Source: CAD feature listing. Evaluate the final solid. Frame: model axes, mm. A direction names the side the tool comes from. Round coordinates to 2 decimals unless told otherwise and drop trailing zeros. Loops run counter-clockwise (first coordinate to the right, second up) from the corner with the lowest first, then second, coordinate; pieces in that order, holes last.
Item 1: First-contact query: P1, Ø1, axis at y = 6, z = -2, coming from the -X side; P2, Ø2, axis at x = 20.5, y = 5, coming from the -Z side; P3, Ø10, axis at x = -63.5, y = 0, coming from the -Z side; P4, Ø1, axis at y = -1, z = 3.5, coming from the +X side. Flat tips, straight axial feed; report the tip coordinate or a pass-through.
Item 2: Section query C-C on x = -6. Return loops of the section in (y, z), then the cut area to 3 significant figures.
Item 3: Section query B-B on y = 3. Give the number of separate pieces and of enclosed holes in the cut face, then the cut area to 3 significant figures.
Item 4: Section query A-A on x = 67.5. Return loops of the section in (y, z), then the cut area to 3 significant figures.
Item 5: Pull-direction query (Y, two-part tool) for faces 3 (the cylindrical face through (-57.54, 1.88, -2.58)), 4 (the flat face through (-1, -12.7, 2)), 5 (the flat face through (-66.8, -5.5, 0)); classes: released by +Y, released by -Y, zero draft, split by the parting line, or undercut.
Item 6: Ray query, L1, parallel to Y at x = -63.5, z = -1.15; L2, parallel to Z at x = -1, y = -2.25; L3, parallel to X at y = 4.25, z = -3.25. Return the intervals inside material, ascending.
Item 7: Access query for faces 1 (the flat face through (1, 12.7, 2)), 2 (the flat face through (16, 0, 0)). Directions: +Z, -Z, +X, -X, +Y, -Y. A direction counts if a zero-diameter tool reaches every point of the face in a straight line with its end or side. Return the directions, or none.
```python
from build123d import *

# Parameters (mm, degrees)
SKETCH1_W                    = 152.4
SKETCH1_H                    = 25.4
BOSS_EXTRUDE1_DEPTH          = 5.08
F_12_5_12_5_DIAMETER_HOLE1_D = 12.5
FILLET3_R                    = 12.7
CUT_EXTRUDE1_START           = -76.2
CUT_EXTRUDE1_OUTLINE_W       = 25.4
CUT_EXTRUDE1_OUTLINE_H       = 2.54
CUT_EXTRUDE1_DEPTH           = 28.395084053
BOSS_EXTRUDE2_START          = -7.62
SKETCH10_R                   = 6.25
BOSS_EXTRUDE2_DEPTH          = 7.62
FILLET12_R                   = 5.08
CUT_EXTRUDE2_START           = -2.54
SKETCH12_R                   = 6.25
CUT_EXTRUDE2_DEPTH           = 2.54
FILLET14_R                   = 5.08
FILLET13_R                   = 5.08
FILLET15_R                   = 5.08


# Read off the part's stored shape, not the designer's step: Cut-Extrude1
with BuildPart() as part:
    # Sketch1 → Boss-Extrude1 (new body)
    with BuildSketch(Plane.XY):
        Rectangle(SKETCH1_W, SKETCH1_H)
    extrude(amount=BOSS_EXTRUDE1_DEPTH)

    # Ø12.5 (12.5) Diameter Hole1 (through all)
    with Locations(Plane.XY.offset(5.08)):
        with Locations((-63.5, 0), (63.5, 0)):
            Hole(F_12_5_12_5_DIAMETER_HOLE1_D / 2)

    # Fillet3
    fillet3_edges = [part.edges().sort_by_distance(p)[0] for p in [
        (-76.2, 12.7, 2.54),
        (-76.2, -12.7, 2.54),
        (76.2, -12.7, 2.54),
        (76.2, 12.7, 2.54),
    ]]
    fillet(fillet3_edges, radius=FILLET3_R - 0.0001)  # a hair under: the kernel refuses the full size

    # Cut-Extrude1 outline → Cut-Extrude1 (cut)
    with BuildSketch(Plane.YZ.offset(CUT_EXTRUDE1_START)):
        with Locations((0, 3.81)):
            Rectangle(CUT_EXTRUDE1_OUTLINE_W, CUT_EXTRUDE1_OUTLINE_H)
    extrude(amount=CUT_EXTRUDE1_DEPTH, mode=Mode.SUBTRACT)

    # Sketch10 → Boss-Extrude2 (add)
    with BuildSketch(Plane.XY.offset(2.54).offset(BOSS_EXTRUDE2_START)):
        with BuildLine():
            Line((-47.804915947, 12.7), (-63.5, 12.7))
            ThreePointArc((-63.5, 12.7), (-72.480256121, 8.980256121), (-76.2, 0))
            ThreePointArc((-76.2, 0), (-72.480256121, -8.980256121), (-63.5, -12.7))
            Line((-63.5, -12.7), (-47.804915947, -12.7))
            Line((-47.804915947, -12.7), (-47.804915947, 12.7))
        make_face()
        with Locations((-63.5, 0)):
            Circle(SKETCH10_R, mode=Mode.SUBTRACT)
    extrude(amount=BOSS_EXTRUDE2_DEPTH)

    # Fillet12
    fillet12_edges = [part.edges().sort_by_distance(p)[0] for p in [
        (-47.804915947, 0, 0),
    ]]
    fillet(fillet12_edges, radius=FILLET12_R - 0.0001)  # a hair under: the kernel refuses the full size

    # Sketch12 → Cut-Extrude2 (cut)
    with BuildSketch(Plane.XY.offset(2.54).offset(CUT_EXTRUDE2_START)):
        with BuildLine():
            Line((-63.5, -12.7), (-47.804915947, -12.7))
            Line((-47.804915947, -12.7), (-47.804915947, 12.7))
            Line((-47.804915947, 12.7), (-63.5, 12.7))
            ThreePointArc((-63.5, 12.7), (-76.2, 0), (-63.5, -12.7))
        make_face()
        with Locations((-63.5, 0)):
            Circle(SKETCH12_R, mode=Mode.SUBTRACT)
    extrude(amount=CUT_EXTRUDE2_DEPTH, mode=Mode.SUBTRACT)


with BuildPart() as cut_extrude2_kept_piece:
    # of the separate pieces the step leaves, the one the design keeps (cut_extrude2_pieces_kept)
    add(part.part.solids().sort_by_distance((-42.725015947, -12.7, 0))[0])

    # Fillet14
    fillet14_edges = [cut_extrude2_kept_piece.edges().sort_by_distance(p)[0] for p in [
        (-47.804915947, 0, 5.08),
    ]]
    fillet(fillet14_edges, radius=FILLET14_R - 0.0001)  # a hair under: the kernel refuses the full size

    # Fillet13
    fillet13_edges = [cut_extrude2_kept_piece.edges().sort_by_distance(p)[0] for p in [
        (-47.804915947, 0, -5.08),
    ]]
    fillet(fillet13_edges, radius=FILLET13_R)

    # Fillet15
    fillet15_edges = [cut_extrude2_kept_piece.edges().sort_by_distance(p)[0] for p in [
        (-47.804915947, 0, 0),
    ]]
    fillet(fillet15_edges, radius=FILLET15_R)


solid = cut_extrude2_kept_piece.part
```
Data:
1. P1: stops at x = -74.95
1. P2: stops at z = 0
1. P3: passes through
1. P4: stops at x = 76.19
2. outline: (-12.7, 0) - (12.7, 0) - (12.7, 5.08) - (-12.7, 5.08) - close
2. area: 129 mm2
3. separate pieces: 3
3. enclosed holes: 0
3. area: 659 mm2
4. outline: (-12.05, 0) - (-4.8, 0) - (-4.8, 5.08) - (-12.05, 5.08) - close; (4.8, 0) - (12.05, 0) - (12.05, 5.08) - (4.8, 5.08) - close
4. area: 73.7 mm2
5. face 3: undercut
5. face 4: released by -Y
5. face 5: zero draft
6. L1: y = -12.7 to -6.25, 6.25 to 12.7
6. L2: z = 0 to 5.08
6. L3: x = -75.47 to -68.08, -58.92 to -47.62
7. face 1: +Z, -Z, +X, -X, +Y
7. face 2: -Z, +X, +Y, -Y
